Part print with two shaded views. Sizes in mm from the minimum x, y, z corner. Give positions to 0.01 mm unless a question says otherwise; leave off trailing zeros. Loops run counter-clockwise (first coordinate to the right, second up) from the corner with the lowest first, then second, coordinate; pieces in that order, holes last. Notation, with made-up numbers: M 24,83.5 L 33,83.5 A20 ccw 33,96.5 Z; hole C 86.25,-18.75 d5. An arc over 180 degrees is marked long. Answer as a JSON object with one key per item and string values. Group by question number.
1. Slice it at B-B (y = 214). List the corners of the cut face in (x, z).
2. Slice it at C-C (x = 3.15). Give the number of separate pieces and of enclosed holes in the cut face, then the cut area to 3 significant figures.
3. Slice it at A-A (z = 6.35). List the corners of the cut face in (x, y) (1 decimal).
4. Slice it at D-D (z = 44.45). List the corners of the cut face in (x, y).
5. Drill centre lines: line 1 along Y through (x, z) = (2.45, 83); line 2 along Y through (x, z) = (0.3, 44); line 3 along Y through (x, z) = (2.9, 56) (1 decimal). Where is each one in solid material? Low to high. Write a range as [from, to].
6. Drop a flat-ended pin along its axis: pin 1 Ø15.5 at (y, z) = (98, 44.45) entering from -X. Give the stop position or say it passes through.
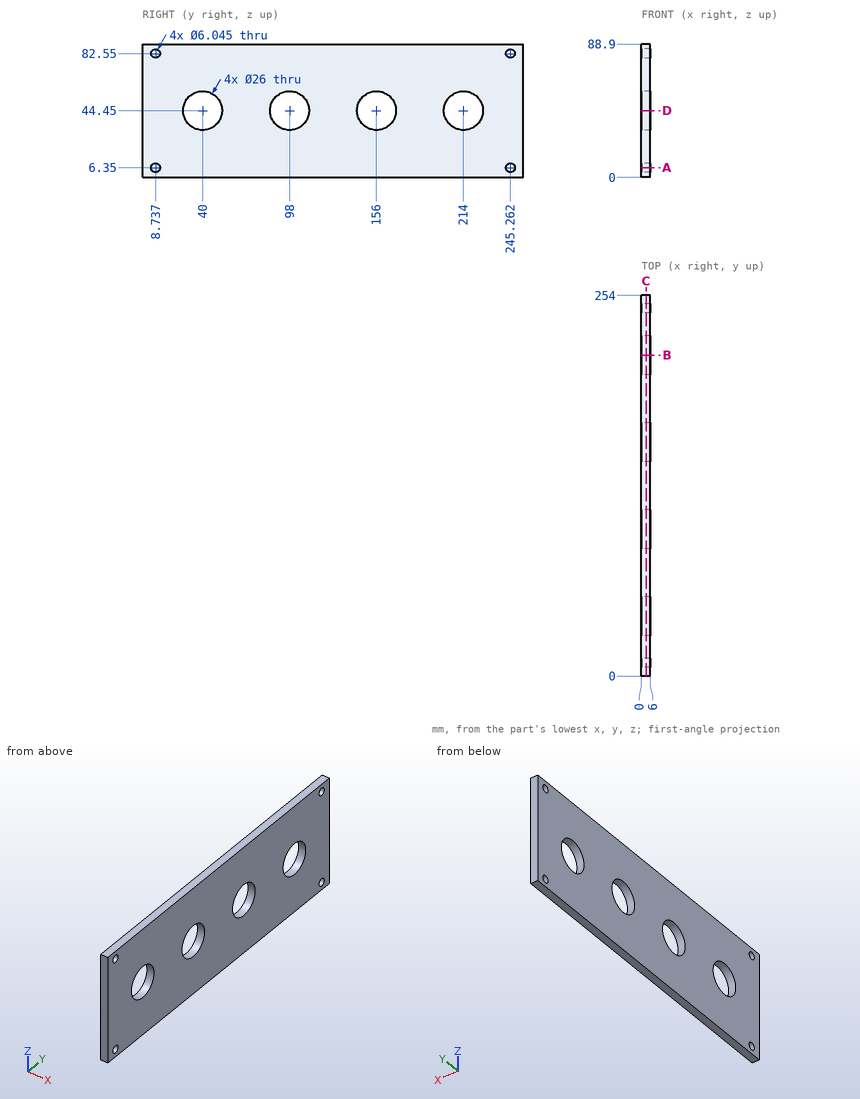
Established:
{
 "1": {"outline": "M 0,0 L 6,0 L 6,31.45 L 0,31.45 Z; M 0,57.45 L 6,57.45 L 6,88.9 L 0,88.9 Z"},
 "2": {"separate pieces": "1", "enclosed holes": "8", "area": "20,300 mm^2"},
 "3": {"outline": "M 0,0 L 6,0 L 6,5.7 L 0,5.7 Z; M 0,11.8 L 6,11.8 L 6,242.2 L 0,242.2 Z; M 0,248.3 L 6,248.3 L 6,254 L 0,254 Z"},
 "4": {"outline": "M 0,0 L 6,0 L 6,27 L 0,27 Z; M 0,53 L 6,53 L 6,85 L 0,85 Z; M 0,111 L 6,111 L 6,143 L 0,143 Z; M 0,169 L 6,169 L 6,201 L 0,201 Z; M 0,227 L 6,227 L 6,254 L 0,254 Z"},
 "5": {"line 1": "y = [0, 5.75], [11.73, 242.27], [248.25, 254]", "line 2": "y = [0, 27.01], [52.99, 85.01], [110.99, 143.01], [168.99, 201.01], [226.99, 254]", "line 3": "y = [0, 34], [46, 92], [104, 150], [162, 208], [220, 254]"},
 "6": {"pin 1": "passes through"}
}
